```python
from build123d import *
from build123d.topology import SkipClean

# Parameters (mm, degrees)
ESQUISSE1_R                  = 20
ESQUISSE1_R_2                = 1.65
BOSS_EXTRU_1_DEPTH           = 8
CONG_1_R                     = 4
ESQUISSE4_R                  = 1.25
ENL_V_MAT_EXTRU_2_DEPTH      = 46
ESQUISSE5_R                  = 1.25
ENL_V_MAT_EXTRU_3_DEPTH      = 46
ENL_V_START                  = -46
ESQUISSE2_R                  = 1.25
ENL_V_MAT_EXTRU_1_DEPTH      = 53
R_P_TITION_CIRCULAIRE1_COUNT = 3
ENL_V_MAT_EXTRU_4_DEPTH      = 2
ENL_V_MAT_EXTRU_5_DEPTH      = 2
R_P_TITION_CIRCULAIRE2_COUNT = 3


with BuildPart() as part:
    # Esquisse1 → Boss.-Extru.1 (new body)
    with BuildSketch(Plane.XY):
        with BuildLine():
            Line((-18.5, 35.99545417), (-18.5, 23.616731357))
            ThreePointArc((-18.5, 23.616731357), (-25.980762114, 15), (-29.70268931, 4.213104291))
            Line((-29.70268931, 4.213104291), (-40.422977732, -1.976257115))
            Line((-40.422977732, -1.976257115), (-37.172977732, -7.605422239))
            Line((-37.172977732, -7.605422239), (-29.8117618, -3.355422239))
            ThreePointArc((-29.8117618, -3.355422239), (-25.980762114, -15), (-17.8117618, -24.14003193))
            Line((-17.8117618, -24.14003193), (-25.172977732, -28.39003193))
            Line((-25.172977732, -28.39003193), (-21.922977732, -34.019197055))
            Line((-21.922977732, -34.019197055), (-11.20268931, -27.829835649))
            ThreePointArc((-11.20268931, -27.829835649), (0, -30), (11.20268931, -27.829835649))
            Line((11.20268931, -27.829835649), (21.922977732, -34.019197055))
            Line((21.922977732, -34.019197055), (25.172977732, -28.39003193))
            Line((25.172977732, -28.39003193), (17.8117618, -24.14003193))
            ThreePointArc((17.8117618, -24.14003193), (25.980762114, -15), (29.8117618, -3.355422239))
            Line((29.8117618, -3.355422239), (37.172977732, -7.605422239))
            Line((37.172977732, -7.605422239), (40.422977732, -1.976257115))
            Line((40.422977732, -1.976257115), (29.70268931, 4.213104291))
            ThreePointArc((29.70268931, 4.213104291), (25.980762114, 15), (18.5, 23.616731357))
            Line((18.5, 23.616731357), (18.5, 35.99545417))
            Line((18.5, 35.99545417), (12, 35.99545417))
            Line((12, 35.99545417), (12, 27.49545417))
            ThreePointArc((12, 27.49545417), (0, 30), (-12, 27.49545417))
            Line((-12, 27.49545417), (-12, 35.99545417))
            Line((-12, 35.99545417), (-18.5, 35.99545417))
        make_face()
        Circle(ESQUISSE1_R, mode=Mode.SUBTRACT)
        with Locations((0, 25)):
            Circle(ESQUISSE1_R_2, mode=Mode.SUBTRACT)
        with Locations((21.650635095, 12.5)):
            Circle(ESQUISSE1_R_2, mode=Mode.SUBTRACT)
        with Locations((21.650635095, -12.5)):
            Circle(ESQUISSE1_R_2, mode=Mode.SUBTRACT)
        with Locations((0, -25)):
            Circle(ESQUISSE1_R_2, mode=Mode.SUBTRACT)
        with Locations((-21.650635095, -12.5)):
            Circle(ESQUISSE1_R_2, mode=Mode.SUBTRACT)
        with Locations((-21.650635095, 12.5)):
            Circle(ESQUISSE1_R_2, mode=Mode.SUBTRACT)
    extrude(amount=BOSS_EXTRU_1_DEPTH)

    # Congé1
    cong_1_edges = [part.edges().sort_by_distance(p)[0] for p in [
        (38.797977732, -4.790839677, 0),
        (38.797977732, -4.790839677, 8),
        (23.547977732, -31.204614493, 0),
        (23.547977732, -31.204614493, 8),
        (15.25, 35.99545417, 0),
        (15.25, 35.99545417, 8),
        (-15.25, 35.99545417, 0),
        (-15.25, 35.99545417, 8),
        (-38.797977732, -4.790839677, 0),
        (-38.797977732, -4.790839677, 8),
        (-23.547977732, -31.204614493, 0),
        (-23.547977732, -31.204614493, 8),
    ]]
    fillet(cong_1_edges, radius=CONG_1_R - 0.0001)  # a hair under: the kernel refuses the full size

    # Esquisse4 → Enlèv. mat.-Extru.2 (cut)
    with BuildSketch(Plane(origin=(9.25, -16.02146997, 0), x_dir=(0.866025403784439, 0.4999999999999994, 0), z_dir=(0.4999999999999994, -0.866025403784439, 0))):
        with Locations((-31.99545417, 4)):
            Circle(ESQUISSE4_R)
    extrude(amount=-ENL_V_MAT_EXTRU_2_DEPTH, mode=Mode.SUBTRACT)

    # Esquisse5 → Enlèv. mat.-Extru.3 (cut)
    with BuildSketch(Plane(origin=(-9.25, -16.02146997, 0), x_dir=(0.8660254037844386, -0.5000000000000002, 0), z_dir=(-0.5000000000000001, -0.8660254037844385, 0))):
        with Locations((31.99545417, 4)):
            Circle(ESQUISSE5_R)
    extrude(amount=-ENL_V_MAT_EXTRU_3_DEPTH, mode=Mode.SUBTRACT)

    # Esquisse7 → Révolution2 (revolve)
    with BuildSketch(Plane.XY.offset(4)):
        with BuildLine():
            Line((-18.5, 35.99545417), (-18.5, 31.99545417))
            Line((-18.5, 31.99545417), (-22.5, 31.99545417))
            ThreePointArc((-22.5, 31.99545417), (-21.328427125, 34.823881294), (-18.5, 35.99545417))
        make_face()
        with BuildLine():
            Line((18.5, 31.99545417), (22.5, 31.99545417))
            ThreePointArc((22.5, 31.99545417), (21.328427125, 34.823881294), (18.5, 35.99545417))
            Line((18.5, 35.99545417), (18.5, 31.99545417))
        make_face()
    r_volution2 = revolve(axis=Axis((-22.5, 31.99545417, 4), (-1, 0, 0)))

    # Esquisse2 → Enlèv. mat.-Extru.1 (cut)
    with BuildSketch(Plane.ZY.offset(18.5).offset(ENL_V_START)):
        with Locations(Location((4, 31.99545417, 0), (0, 0, 90))):
            Circle(ESQUISSE2_R)
    enl_v_mat_extru_1 = extrude(amount=ENL_V_MAT_EXTRU_1_DEPTH, mode=Mode.SUBTRACT)

    # Répétition circulaire1: Révolution2, Enlèv. mat.-Extru.1 ×3 about axis
    with SkipClean():  # the faces are left unmerged after this step: merging them gives an invalid solid
        r_p_tition_circulaire1_axis = Axis((0, 0, 0), (0, 0, 1))
        add([r_volution2.rotate(r_p_tition_circulaire1_axis, i * 360 / R_P_TITION_CIRCULAIRE1_COUNT) for i in range(1, R_P_TITION_CIRCULAIRE1_COUNT)])
        add([enl_v_mat_extru_1.rotate(r_p_tition_circulaire1_axis, i * 360 / R_P_TITION_CIRCULAIRE1_COUNT) for i in range(1, R_P_TITION_CIRCULAIRE1_COUNT)], mode=Mode.SUBTRACT)

    # Esquisse8 → Enlèv. mat.-Extru.4 (cut)
    with SkipClean():  # the faces are left unmerged after this step: merging them gives an invalid solid
        with BuildSketch(Plane(origin=(-12, 0, 0), x_dir=(0, 0, -1), z_dir=(1, 0, 0))):
            Polygon((-0.535898385, 31.99545417), (-2.267949192, 34.99545417), (-5.732050808, 34.99545417), (-7.464101615, 31.99545417), (-5.732050808, 28.99545417), (-2.267949192, 28.99545417), align=None)
        enl_v_mat_extru_4 = extrude(amount=-ENL_V_MAT_EXTRU_4_DEPTH, mode=Mode.SUBTRACT)

    # Esquisse9 → Enlèv. mat.-Extru.5 (cut)
    with SkipClean():  # the faces are left unmerged after this step: merging them gives an invalid solid
        with BuildSketch(Plane.ZY.offset(-12)):
            Polygon((0.535898385, 31.99545417), (2.267949192, 28.99545417), (5.732050808, 28.99545417), (7.464101615, 31.99545417), (5.732050808, 34.99545417), (2.267949192, 34.99545417), align=None)
        enl_v_mat_extru_5 = extrude(amount=-ENL_V_MAT_EXTRU_5_DEPTH, mode=Mode.SUBTRACT)

    # Répétition circulaire2: Enlèv. mat.-Extru.4, Enlèv. mat.-Extru.5 ×3 about axis
    with SkipClean():  # the faces are left unmerged after this step: merging them gives an invalid solid
        r_p_tition_circulaire2_axis = Axis((0, 0, 0), (0, 0, 1))
        add([enl_v_mat_extru_4.rotate(r_p_tition_circulaire2_axis, i * 360 / R_P_TITION_CIRCULAIRE2_COUNT) for i in range(1, R_P_TITION_CIRCULAIRE2_COUNT)], mode=Mode.SUBTRACT)
        add([enl_v_mat_extru_5.rotate(r_p_tition_circulaire2_axis, i * 360 / R_P_TITION_CIRCULAIRE2_COUNT) for i in range(1, R_P_TITION_CIRCULAIRE2_COUNT)], mode=Mode.SUBTRACT)


solid = part.part
```
Here's how the part is built. I have some questions about the finished solid (model axes, mm). A direction names the side the tool comes from. Round coordinates to 2 decimals unless told otherwise and drop trailing zeros. Order: outer loops, then holes, each group sorted by start corner. A loop starts at its lowest first (then second) coordinate and runs counter-clockwise, first axis right, second up. Notation, with made-up numbers: M -18,45 L 35,45 A7 ccw 35,52 Z; hole C -24,18.25 d9. An arc over 180 degrees is marked long. Answer as CSV lines item,"result".
Item 1: Please list where these lines run through material, in increasing order: L1, parallel to X at y = -32.5, z = 5; L2, parallel to Y at x = -18, z = 2; L3, parallel to Y at x = 18, z = 3.75. Write a range as [from, to].
From the geometry:
L1,"[-22.65, -19.05], [-17.32, -14.62], [14.62, 17.32], [19.05, 22.65]"
L2,"[-35.45, -24.25], [-24, -8.72], [8.72, 35.46]"
L3,"[-35.98, -35.26], [-30.36, -24.25], [-24, -8.72], [8.72, 30.77], [33.22, 35.99]"
Item 2: Imagine slicing it at B-B on y = 12.5. List the corners of the cut face in (x, z) for me, and give its area (3 significant figures).
From the geometry:
outline,"M -27.27,0 L -23.3,0 L -23.3,8 L -27.27,8 Z; M -20,0 L -15.61,0 L -15.61,8 L -20,8 Z; M 15.61,0 L 20,0 L 20,8 L 15.61,8 Z; M 23.3,0 L 27.27,0 L 27.27,8 L 23.3,8 Z"
area,"134 mm2"
Item 3: Imagine slicing it at C-C on x = -5.5. List the corners of the cut face in (y, z) for me, and give its area (3 significant figures).
From the geometry:
outline,"M -29.49,0 L -19.23,0 L -19.23,8 L -29.49,8 Z; M 19.23,0 L 29.49,0 L 29.49,8 L 19.23,8 Z"
area,"164 mm2"
Item 4: Which directions (+Z, -Z, +X, -X, +Y, -Y) give clear straight access to the entire face, cutting with the end or side of a thin tool? Please do faces 4 (the cylindrical face through (-22.537, -30.674, 1.203)), 5 (the flat face through (-31.604, -3.252, 3.976)), 6 (the flat face through (18.62, -25.74, 3.98)), 7 (the cylindrical face through (-0.215, 26.636, 3.944)), 8 (the flat face through (-20.745, -28.143, 2.509)).
From the geometry:
face 4,"-Z, -X, -Y"
face 5,"-Y"
face 6,"+X"
face 7,"+Z, -Z"
face 8,"none"
Item 5: We'd pull the mould along Z, two halves only. Please class faces 1 (the flat face through (-1, -21, 0)), 2 (the cylindrical face through (-4.336, -19.524, 3.944)), 3 (the flat face through (-19.94, -26.5, 6.61)): +Z half, -Z half, draft (parallel to the pull), parting line (faces both ways), or undercut.
From the geometry:
face 1,"-Z half"
face 2,"draft"
face 3,"undercut"
Item 6: Imagine slicing it at A-A on x = 13. Give the number of separate pieces and of enclosed holes in the cut face, and give its area (3 significant figures).
From the geometry:
separate pieces,"2"
enclosed holes,"1"
area,"238 mm2"
Item 7: For pin 1 (2.5 mm diameter, centred on y = 28.5, z = 4.5, fed in from +X); pin 2 (2 mm diameter, centred on x = -12.5, z = 4, fed in from -Y); pin 3 (4 mm diameter, centred on y = 30, z = 5.5, fed in from -X); pin 4 (2 mm diameter, centred on y = 32, z = 4, fed in from +X), each with a flat end and sliding along its axis, tell me the tip position at first contact or that it passes through.
From the geometry:
pin 1,"x = 21.79"
pin 2,"y = -29.16"
pin 3,"x = -22.3"
pin 4,"through"
